Design review of the part built by this model. Coordinates are the model's own, in mm. Face numbers are marked on the shaded views. A direction names the side the tool comes from. Give positions to 0.01 mm unless a question says otherwise; leave off trailing zeros. Write each loop counter-clockwise with the first axis right and the second up, starting at its lowest first coordinate (ties: lowest second). Pieces come first, ordered by that corner, then holes. Notation, with made-up numbers: M 86,-16.75 L 111,-16.75 A24 cw 111,14.25 Z; hole C 50.25,-18 d5. An arc over 180 degrees is marked long. Use a Markdown table: item, result. Add a question column.
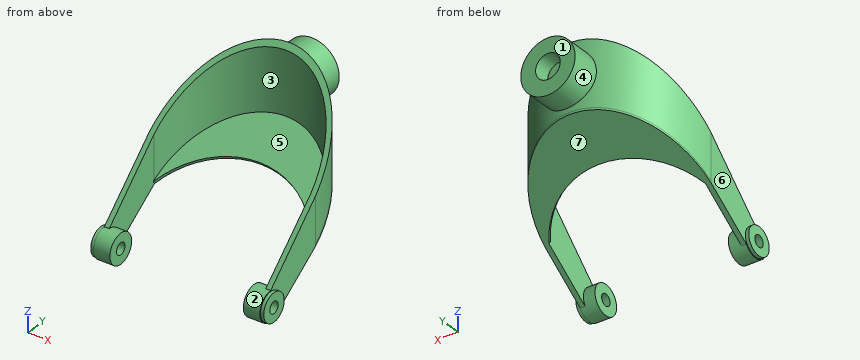
```python
from build123d import *

# Parameters (mm, degrees)
SALIENTE_EXTRUIR1_DEPTH = 100
CORTAR_EXTRUIR1_DEPTH   = 141
CROQUIS3_R              = 9
SALIENTE_EXTRUIR2_DEPTH = 10
CROQUIS4_R              = 8.5
SALIENTE_EXTRUIR3_DEPTH = 2
CROQUIS5_R              = 3.5
CORTAR_EXTRUIR2_DEPTH   = 14
SALIENTE_EXTRUIR5_DEPTH = 1
SALIENTE_EXTRUIR7_REACH = 157.144
CROQUIS11_R             = 16.5
SALIENTE_EXTRUIR8_START = 15
CROQUIS12_R             = 16.5
SALIENTE_EXTRUIR8_DEPTH = 15
CROQUIS13_R             = 7.5
CORTAR_EXTRUIR5_DEPTH   = 10
CORTAR_EXTRUIR6_START   = 24.949967
CORTAR_EXTRUIR6_DEPTH   = 35.050033
SALIENTE_EXTRUIR9_REACH = 151.051
CROQUIS17_W             = 3
CROQUIS17_H             = 1


with BuildPart() as part:
    # Croquis1 → Saliente-Extruir1 (new body)
    with BuildSketch(Plane.XY):
        with BuildLine():
            Line((69.641072198, 46.543110775), (69.641072198, -23.536729858))
            Line((69.641072198, -23.536729858), (66.641072198, -23.536729858))
            Line((66.641072198, -23.536729858), (66.641072198, 46.463270142))
            ThreePointArc((66.641072198, 46.463270142), (19.141072198, 91.463270142), (-28.358927802, 46.463270142))
            Line((-28.358927802, 46.463270142), (-28.358927802, -23.536729858))
            Line((-28.358927802, -23.536729858), (-31.358927802, -23.536729858))
            Line((-31.358927802, -23.536729858), (-31.358927802, 46.543110775))
            ThreePointArc((-31.358927802, 46.543110775), (19.141072198, 94.463270142), (69.641072198, 46.543110775))
        make_face()
    extrude(amount=SALIENTE_EXTRUIR1_DEPTH)

    # Croquis2 → Cortar-Extruir1 (cut)
    with BuildSketch(Plane(origin=(69.641072198, 0, 0), x_dir=(0, 0, -1), z_dir=(1, 0, 0))):
        Polygon((-100, 94.463270142), (-18, 9.463270142), (0, 9.463270142), (-60, 94.463270142), (0, 94.463270142), (15.172467856, 86.125033525), (0, 6.963270142), (0, -23.536729858), (-100, -23.536729858), align=None)
    extrude(amount=-CORTAR_EXTRUIR1_DEPTH, mode=Mode.SUBTRACT)

    # Croquis3 → Saliente-Extruir2 (add)
    with BuildSketch(Plane(origin=(69.641072198, 0, 0), x_dir=(0, 0, -1), z_dir=(1, 0, 0))):
        with Locations(Location((-9, 9.463270142, 0), (0, 0, 90))):
            Circle(CROQUIS3_R)
    saliente_extruir2 = extrude(amount=-SALIENTE_EXTRUIR2_DEPTH)

    # Croquis4 → Saliente-Extruir3 (add)
    with BuildSketch(Plane(origin=(69.641072198, 0, 0), x_dir=(0, 0, -1), z_dir=(1, 0, 0))):
        with Locations(Location((-9, 9.463270142, 0), (0, 0, 270))):
            Circle(CROQUIS4_R)
    saliente_extruir3 = extrude(amount=SALIENTE_EXTRUIR3_DEPTH)

    # Croquis5 → Cortar-Extruir2 (cut)
    with BuildSketch(Plane(origin=(71.641072198, 0, 0), x_dir=(0, 0, -1), z_dir=(1, 0, 0))):
        with Locations(Location((-9, 9.463270142, 0), (0, 0, 90))):
            Circle(CROQUIS5_R)
    cortar_extruir2 = extrude(amount=-CORTAR_EXTRUIR2_DEPTH, mode=Mode.SUBTRACT)

    # Simetría1: Saliente-Extruir2, Saliente-Extruir3, Cortar-Extruir2 across plane
    add(saliente_extruir2.mirror(Plane(origin=(19.141072198, 0, 0), x_dir=(0, 0, 1), z_dir=(1, 0, 0))))
    add(saliente_extruir3.mirror(Plane(origin=(19.141072198, 0, 0), x_dir=(0, 0, 1), z_dir=(1, 0, 0))))
    add(cortar_extruir2.mirror(Plane(origin=(19.141072198, 0, 0), x_dir=(0, 0, 1), z_dir=(1, 0, 0))), mode=Mode.SUBTRACT)

    # Croquis6 → Saliente-Extruir5 (add, symmetric)
    with BuildSketch(Plane(origin=(0, 3.147138338, -4.458445979), x_dir=(-1, 0, 0), z_dir=(0, 0.5766831975986554, -0.8169678632647617))):
        with BuildLine():
            Line((-67.534417906, 18.111485144), (-66.641072198, 18.111485144))
            Line((-66.641072198, 18.111485144), (-66.641072198, 53.020606748))
            add(Edge.make_bspline(
                [(-19.141072198, 108.102332754), (-64.206861672, 108.102332754), (-66.641072198, 53.020606748)],
                knots=[3.141592654, 3.141592654, 3.141592654, 4.658348082, 4.658348082, 4.658348082], degree=2, weights=[1, 0.725952684, 1]))
            Line((-19.141072198, 108.102332754), (-19.141072198, 111.774447821))
            add(Edge.make_bspline(
                [(-19.141072198, 111.774447821), (-67.127128374, 111.774447821), (-69.641072198, 53.118334745)],
                knots=[3.141592654, 3.141592654, 3.141592654, 4.659975938, 4.659975938, 4.659975938], degree=2, weights=[1, 0.725392669, 1]))
            Line((-69.641072198, 53.118334745), (-69.641072198, 18.111485144))
            Line((-69.641072198, 18.111485144), (-67.534417906, 18.111485144))
        make_face()
        with BuildLine():
            Line((-19.141072198, 111.774447821), (-19.141072198, 108.102332754))
            add(Edge.make_bspline(
                [(28.358927802, 53.020606748), (25.924717276, 108.102332754), (-19.141072198, 108.102332754)],
                knots=[1.624837225, 1.624837225, 1.624837225, 3.141592654, 3.141592654, 3.141592654], degree=2, weights=[1, 0.725952684, 1]))
            Line((28.358927802, 53.020606748), (28.358927802, 18.111485144))
            Line((28.358927802, 18.111485144), (31.358927802, 18.111485144))
            Line((31.358927802, 18.111485144), (31.358927802, 53.118334745))
            add(Edge.make_bspline(
                [(31.358927802, 53.118334745), (28.844983978, 111.774447821), (-19.141072198, 111.774447821)],
                knots=[1.62320937, 1.62320937, 1.62320937, 3.141592654, 3.141592654, 3.141592654], degree=2, weights=[1, 0.725392669, 1]))
        make_face()
        with BuildLine():
            add(Edge.make_bspline(
                [(-19.141072198, 108.102332754), (-64.206861672, 108.102332754), (-66.641072198, 53.020606748)],
                knots=[3.141592654, 3.141592654, 3.141592654, 4.658348082, 4.658348082, 4.658348082], degree=2, weights=[1, 0.725952684, 1]))
            ThreePointArc((-66.641072198, 53.020606748), (-46.903607099, 74.026047186), (-19.141072198, 81.774447821))
            Line((-19.141072198, 81.774447821), (-19.141072198, 108.102332754))
        make_face()
        with BuildLine():
            Line((-19.141072198, 108.102332754), (-19.141072198, 81.774447821))
            ThreePointArc((-19.141072198, 81.774447821), (8.621462703, 74.026047186), (28.358927802, 53.020606748))
            add(Edge.make_bspline(
                [(28.358927802, 53.020606748), (25.924717276, 108.102332754), (-19.141072198, 108.102332754)],
                knots=[1.624837225, 1.624837225, 1.624837225, 3.141592654, 3.141592654, 3.141592654], degree=2, weights=[1, 0.725952684, 1]))
        make_face()
    extrude(amount=SALIENTE_EXTRUIR5_DEPTH, both=True)

    # Croquis11 → Saliente-Extruir7 (add, up to next)
    with BuildSketch(Plane(origin=(0, 95, 0), x_dir=(1, 0, 0), z_dir=(0, 1, 0)), mode=Mode.PRIVATE) as saliente_extruir7_sk1:
        with Locations(Location((21.175045512, -79.353799607, 0), (0, 0, 270))):
            Circle(CROQUIS11_R)
    saliente_extruir7_tool1 = extrude(saliente_extruir7_sk1.sketch, amount=-SALIENTE_EXTRUIR7_REACH, mode=Mode.PRIVATE) - part.part
    add(saliente_extruir7_tool1.solids().sort_by_distance((21.175046, 95, 79.3538))[0])

    # Croquis12 → Saliente-Extruir8 (add)
    with BuildSketch(Plane(origin=(0, 95, 0), x_dir=(1, 0, 0), z_dir=(0, 1, 0)).offset(SALIENTE_EXTRUIR8_START)):
        with Locations(Location((21.175045512, -79.353799607, 0), (0, 0, 270))):
            Circle(CROQUIS12_R)
    extrude(amount=-SALIENTE_EXTRUIR8_DEPTH)

    # Croquis13 → Cortar-Extruir5 (cut)
    with BuildSketch(Plane(origin=(0, 110, 0), x_dir=(1, 0, 0), z_dir=(0, 1, 0))):
        with Locations(Location((21.175045512, -79.353799607, 0), (0, 0, 270))):
            Circle(CROQUIS13_R)
    extrude(amount=-CORTAR_EXTRUIR5_DEPTH, mode=Mode.SUBTRACT)

    # Croquis8 → Cortar-Extruir6 (cut)
    with BuildSketch(Plane.XY.offset(CORTAR_EXTRUIR6_START)):
        with BuildLine():
            Line((-31.358927802, 46.543110775), (-43.995227874, 50.405646303))
            Line((-43.995227874, 50.405646303), (-32.93588468, 104.800400399))
            Line((-32.93588468, 104.800400399), (86.326861303, 97.464379117))
            Line((86.326861303, 97.464379117), (84.859657046, 44.645025888))
            Line((84.859657046, 44.645025888), (69.641072198, 46.543110775))
            ThreePointArc((69.641072198, 46.543110775), (19.141072198, 94.463270142), (-31.358927802, 46.543110775))
        make_face()
    extrude(amount=CORTAR_EXTRUIR6_DEPTH, mode=Mode.SUBTRACT)

    # Croquis17 → Saliente-Extruir9 (add, up to next)
    with BuildSketch(Plane(origin=(0, 14.796501319, 10.444589166), x_dir=(1, 0, 0), z_dir=(0, -0.8169678632647617, -0.5766831975986554)), mode=Mode.PRIVATE) as saliente_extruir9_sk1:
        with Locations((-29.858927802, -5.957308885)):
            Rectangle(CROQUIS17_W, CROQUIS17_H)
    saliente_extruir9_tool1 = extrude(saliente_extruir9_sk1.sketch, amount=SALIENTE_EXTRUIR9_REACH, mode=Mode.PRIVATE) - part.part
    saliente_extruir9 = saliente_extruir9_tool1.solids().sort_by_distance((-29.858928, 18.231981, 5.577659))[0]
    add(saliente_extruir9)

    # Simetría2: Saliente-Extruir9 across plane
    add(saliente_extruir9.mirror(Plane(origin=(19.141072198, 0, 0), x_dir=(0, 0, 1), z_dir=(1, 0, 0))))


solid = part.part
```
(1) Machinability: for the marked faces 1, 2 and 3, which of the approach directions +Z, -Z, +X, -X, +Y, -Y give a long, thin tool a straight path to every point of the face, cutting with its end or side? Answer none if there is none.
(2) Add section D-D on x = 9. Give the boundary of the cut face in (y, z).
(3) Wall thickness on L1, parallel to Y at x = -27, z = 9; L2, parallel to X at y = 85, z = 70; L3, parallel to X at y = 102.5, z = 78: over which ranges is each line inside the solid? List them lowest first.
(4) For pin 1 (8 mm diameter, centred on y = 25.5, z = 30, fed in from +X); pin 2 (8 mm diameter, centred on x = -16.5, z = 89, fed in from +Y); pin 3 (3 mm diameter, centred on x = 40, z = 74, fed in from +Y); pin 4 (6.5 mm diameter, centred on y = 9.46, z = 9, fed in from -X), all flat-tipped, find the tip position at first contact; note any pin that passes through.
(5) Add section A-A on x = 64. Give the boundary of the cut face in (y, z), then the cut area to 3 significant figures.
(6) The part is to be moulded in two halves that separate along X. For the marked faces 4, 5, 6 and 7, say which applies: released by +X, released by -X, zero draft, split by the parting line, or undercut.
(7) Add section B-B on z = 9. Give the boundary of the cut face in (x, y).
(8) Add section C-C on y = 27. Give the boundary of the cut face in (x, z), then the cut area to 3 significant figures.
From the geometry:
| question | item | result |
|---|---|---|
| 1 | face 1 | +Z, -Z, +X, -X, +Y |
| 1 | face 2 | none |
| 1 | face 3 | +Z, -Y |
| 2 | outline | M 68.59,42.96 L 69.74,41.32 L 93.44,58.05 L 93.44,68.22 L 110,68.22 L 110,90.49 L 93.44,90.49 L 93.44,99.01 L 90.37,96.05 L 90.37,58.33 Z |
| 3 | L1 | y = 0.46 to 5.96, 12.96 to 18.46 |
| 3 | L2 | x = -10.31 to -4.8, 43.08 to 48.6 |
| 3 | L3 | x = 4.73 to 13.8, 28.55 to 37.62 |
| 4 | pin 1 | stops at x = 69.64 |
| 4 | pin 2 | stops at y = 83.34 |
| 4 | pin 3 | stops at y = 90.61 |
| 4 | pin 4 | passes through |
| 5 | outline | C 9.46,9 d18; M 49.56,29.53 L 50.72,27.9 L 67.24,39.56 L 67.24,73.74 L 59.72,66.48 L 59.72,36.7 Z; hole C 9.46,9 d7 |
| 5 | area | 489 mm^2 |
| 6 | face 4 | split by the parting line |
| 6 | face 5 | undercut |
| 6 | face 6 | released by -X |
| 6 | face 7 | zero draft |
| 7 | outline | M -33.36,0.96 L -31.36,0.96 L -31.36,0.46 L -21.36,0.46 L -21.36,5.96 L -33.36,5.96 Z; M -33.36,12.96 L -21.36,12.96 L -21.36,18.46 L -28.36,18.46 L -28.36,23.95 L -31.36,23.95 L -31.36,17.96 L -33.36,17.96 Z; M 59.64,0.46 L 69.64,0.46 L 69.64,0.96 L 71.64,0.96 L 71.64,5.96 L 59.64,5.96 Z; M 59.64,12.96 L 71.64,12.96 L 71.64,17.96 L 69.64,17.96 L 69.64,23.95 L 66.64,23.95 L 66.64,18.46 L 59.64,18.46 Z |
| 8 | outline | M -31.36,11.15 L -28.36,11.15 L -28.36,34.92 L -31.36,34.92 Z; M 66.64,11.15 L 69.64,11.15 L 69.64,34.92 L 66.64,34.92 Z |
| 8 | area | 143 mm^2 |
